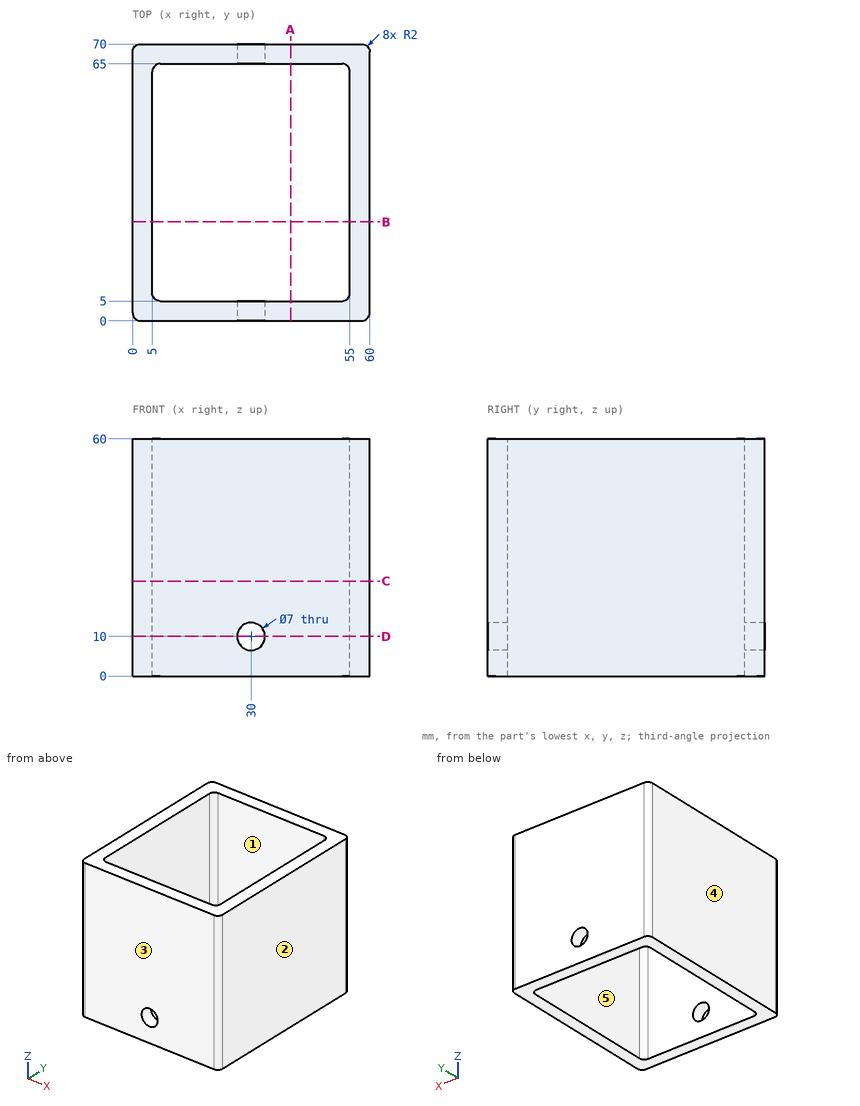
Verification items for this drawing (mm, ordinates from the low corner). A direction names the side the tool comes from. Round coordinates to 2 decimals unless told otherwise and drop trailing zeros. Loops run counter-clockwise (first coordinate to the right, second up) from the corner with the lowest first, then second, coordinate; pieces in that order, holes last. Notation, with made-up numbers: (64.25, 31.5) - (86.25, 31.5) arc R17 cw to (86.25, 35.5) - close; hole circle Ø9 at (-32.5, 68.5). An arc over 180 degrees is marked (long way). Answer as CSV lines item,"result". Start each with the question number.
Item 1: Section check B-B (y = 25). Record the boundary of the cut face in (x, z).
Item 2: Scan lines: line 1 (Z direction, x = 30, y = 3.4); line 2 (Y direction, x = 15, z = 10.5); line 3 (X direction, y = 8.5, z = 24.5). Record each from-to range of solid material in increasing order. Write a range as [from, to].
Item 3: Section check C-C (z = 24). Record the boundary of the cut face in (x, y).
Item 4: Set-up check for the marked faces 1 and 2: record each of +Z, -Z, +X, -X, +Y, -Y from which the full face is reachable in a straight line by a thin tool's end or side.
Item 5: Section check A-A (x = 40). Record the boundary of the cut face in (y, z).
Item 6: Section check D-D (z = 10). Record the boundary of the cut face in (x, y).
Item 7: Release check for a two-part mould opening along Y. For the marked faces 3, 4 and 5 record: +Y half, -Y half, draft (parallel to the pull), parting line (faces both ways), or undercut.
Report:
1,outline,"(0, 0) - (5, 0) - (5, 60) - (0, 60) - close; (55, 0) - (60, 0) - (60, 60) - (55, 60) - close"
2,line 1,"z = [0, 6.5], [13.5, 60]"
2,line 2,"y = [0, 5], [65, 70]"
2,line 3,"x = [0, 5], [55, 60]"
3,outline,"(0, 2) arc R2 ccw to (2, 0) - (58, 0) arc R2 ccw to (60, 2) - (60, 68) arc R2 ccw to (58, 70) - (2, 70) arc R2 ccw to (0, 68) - close; hole (5, 7) arc R2 ccw to (7, 5) - (53, 5) arc R2 ccw to (55, 7) - (55, 63) arc R2 ccw to (53, 65) - (7, 65) arc R2 ccw to (5, 63) - close"
4,face 1,"+Z, -Z"
4,face 2,"+Z, -Z, +X, +Y, -Y"
5,outline,"(0, 0) - (5, 0) - (5, 60) - (0, 60) - close; (65, 0) - (70, 0) - (70, 60) - (65, 60) - close"
6,outline,"(0, 2) arc R2 ccw to (2, 0) - (26.5, 0) - (26.5, 5) - (7, 5) arc R2 cw to (5, 7) - (5, 63) arc R2 cw to (7, 65) - (26.5, 65) - (26.5, 70) - (2, 70) arc R2 ccw to (0, 68) - close; (33.5, 0) - (58, 0) arc R2 ccw to (60, 2) - (60, 68) arc R2 ccw to (58, 70) - (33.5, 70) - (33.5, 65) - (53, 65) arc R2 cw to (55, 63) - (55, 7) arc R2 cw to (53, 5) - (33.5, 5) - close"
7,face 3,"-Y half"
7,face 4,"draft"
7,face 5,"undercut"
